CAD build for the part. Positions are in the model's coordinates, mm. A direction names the side the tool comes from. Give positions to 0.01 mm unless a question says otherwise; leave off trailing zeros. Loops run counter-clockwise (first coordinate to the right, second up) from the corner with the lowest first, then second, coordinate; pieces in that order, holes last.
Item 1: Probe probe 1 along Z at (x, y) = (-1.3, 0.3); probe 2 along Z at (x, y) = (-0.9, -1.3); probe 3 along X at (y, z) = (1.4, 1). List the from-to ranges inside material, lowest first.
Item 2: Which spindle directions (+Z, -Z, +X, -X, +Y, -Y) get a long thin tool onto all of the face, cutting with end or side? Do faces 1 (the cylindrical face through (-0.54, 2.44, 2.47)), 2 (the cylindrical face through (1.5, -0.07, -0.99)), 3 (the flat face through (1, -1, 5)). Say none if no direction does.
Item 3: Saw through at D-D on z = 6.5. Give the cut face in (x, y), plus the area to 3 significant figures.
Item 4: Drop flat-ended pins along their axis: P1, Ø1, axis at x = -1.5, z = 2.5, coming from the -Y side; P2, Ø1, axis at x = 1.5, z = 5, coming from the +Y side. Give the stop position or say it passes through.
Item 5: Saw through at A-A on x = 0. Give the cut face in (y, z).
Item 6: Saw through at C-C on z = 1.75. Give the cut face in (x, y).
Autodesk Inventor part; units mm, degrees
ref_plane "YZ Plane" through (0, 0, 0) normal (1, 0, 0) x (0, 1, 0)
ref_plane "XZ Plane" through (0, 0, 0) normal (0, 1, 0) x (-1, 0, 0)
ref_plane "XY Plane" through (0, 0, 0) normal (0, 0, 1) x (1, 0, 0)
sketch "スケッチ1" plane through (0, 0, 0) normal (0, 0, 1) x (1, 0, 0)
  circle A0 centre (0, 0) radius 2.5
  dimension "d10" = 5
extrude "押し出し1" add sketch "スケッチ1" along normal blind 5
sketch "スケッチ2" plane through (0, 0, 5) normal (0, 0, 1) x (1, 0, 0)
  circle A0 centre (0, 0) radius 1.2
  dimension "d7" = 2.4
extrude "押し出し2" add sketch "スケッチ2" along normal blind 2
fillet "フィレット1" radius 0.5 2 edges at (-2.5, 0, 5) (-2.5, 0, 0)
sketch "スケッチ3" plane through (0, 0, 0) normal (0, 0, -1) x (-1, 0, 0)
  circle A0 centre (0, 0) radius 2
  circle A1 centre (0, 0) radius 1.5
  dimension "d12" = 3
extrude "押し出し3" add sketch "スケッチ3" along normal blind 2 contours A1
properties part number "worka"
Results below:
1. probe 1: z = -2 to 5
1. probe 2: z = 0 to 5
1. probe 3: x = -2.07 to 2.07
2. face 1: +Z, -Z
2. face 2: -Z
2. face 3: +Z
3. outline: circle Ø2.4 at (0, 0)
3. area: 4.52 mm2
4. P1: stops at y = -2.29
4. P2: stops at y = 2.2
5. outline: (-2.5, 0.5) arc R0.5 ccw to (-2, 0) - (-1.5, 0) - (-1.5, -2) - (1.5, -2) - (1.5, 0) - (2, 0) arc R0.5 ccw to (2.5, 0.5) - (2.5, 4.5) arc R0.5 ccw to (2, 5) - (1.2, 5) - (1.2, 7) - (-1.2, 7) - (-1.2, 5) - (-2, 5) arc R0.5 ccw to (-2.5, 4.5) - close
6. outline: circle Ø5 at (0, 0)
